Autodesk Fusion 360 part; units mm, degrees
sketch "Sketch1" plane through (0, 0, 0) normal (1, 0, 0) x (0, 1, 0) in component "latch_shuttle"
  arc A0 (-8.3077, 5.5575) -> (-1.6746, 2.5672) centre (9.4182, 36.0259) ccw
  arc A1 (-8.3077, 5.5575) -> (-9.6608, 5.2196) centre (-8.8106, 4.6931) ccw
  line L0 (-12.0836, 1.3076) -> (-9.6608, 5.2196)
  arc A2 (-12.0836, 1.3076) -> (-11.739, -0.0818) centre (-11.2334, 0.781) ccw
  arc A3 (-11.739, -0.0818) -> (-10.3245, -0.8742) centre (9.4182, 36.0259) ccw
  arc A4 (-10.3245, -0.8742) -> (-9.5002, -0.6041) centre (-10.0414, -0.3452) ccw
  line L1 (-9.5002, -0.6041) -> (-8.9235, 0.6015)
  arc A5 (-5.6086, 0.4414) -> (-8.9235, 0.6015) centre (-7.2997, -0.1753) ccw
  line L2 (-5.6086, 0.4414) -> (-4.4802, -2.6531)
  arc A6 (-4.4802, -2.6531) -> (-3.2044, -3.8747) centre (-2.6012, -1.9679) ccw
  arc A7 (-3.2044, -3.8747) -> (7.5742, -5.7831) centre (9.4182, 36.0259) ccw
  arc A8 (7.5742, -5.7831) -> (8.6182, -4.784) centre (7.6182, -4.784) ccw
  line L3 (8.6182, 3.9982) -> (8.6182, -4.784)
  arc A9 (8.6182, 3.9982) -> (7.6743, 4.9966) centre (7.6182, 3.9982) ccw
  arc A10 (5.7512, 5.1647) -> (7.6743, 4.9966) centre (9.4182, 36.0259) ccw
  arc A11 (5.7512, 5.1647) -> (4.8102, 4.7397) centre (5.6332, 4.1717) ccw
  arc A12 (-1.6746, 2.5672) -> (4.8102, 4.7397) centre (0.1191, 7.9776) ccw
extrude "Extrude1" add sketch "Sketch1" along normal mid plane 10.6 in component "latch_shuttle"
chamfer "Chamfer1" distance 0.4 angle 45 34 edges at (5.3, -5.0685, 3.8907) (5.3, -9.0529, 5.6633) (5.3, -10.8722, 3.2636) (5.3, -12.204, 0.5403) (5.3, -11.0356, -0.4848) (5.3, -9.8546, -0.9153) (5.3, -9.2118, -0.0013) (5.3, -7.2129, 1.6226) (5.3, -5.0444, -1.1058) (5.3, -3.9845, -3.4124) (5.3, 2.1222, -5.1828) (5.3, 8.3096, -5.5066) (5.3, 8.6182, -0.3929) (5.3, 8.3449, 4.6851) (5.3, 6.7115, 5.0657) (5.3, 5.2216, 5.0831) (5.3, 1.9298, 2.5728) (-5.3, 8.6182, -0.3929) (-5.3, 8.3096, -5.5066) (-5.3, 2.1222, -5.1828) (-5.3, -3.9845, -3.4124) (-5.3, -5.0444, -1.1058) (-5.3, -7.2129, 1.6226) (-5.3, -9.2118, -0.0013) (-5.3, -9.8546, -0.9153) (-5.3, -11.0356, -0.4848) (-5.3, -12.204, 0.5403) (-5.3, -10.8722, 3.2636) (-5.3, -9.0529, 5.6633) (-5.3, -5.0685, 3.8907) (-5.3, 1.9298, 2.5728) (-5.3, 5.2216, 5.0831) (-5.3, 6.7115, 5.0657) (-5.3, 8.3449, 4.6851) in component "latch_shuttle"
sketch "Sketch2" plane through (0, 8.6182, 0) normal (0, 1, 0) x (-1, 0, 0) in component "latch_shuttle"
  line L0 (4.9, -4.784) -> (4.9, 3.9982)
  line L1 (4.9, 3.9982) -> (-4.9, 3.9982)
  line L2 (-4.9, 3.9982) -> (-4.9, -4.784)
  line L3 (-4.9, -4.784) -> (4.9, -4.784)
  circle A0 centre (0, -0.4177) radius 1.6
  circle A1 centre (0, -0.4177) radius 2.35
extrude "Extrude2" cut sketch "Sketch2" against normal blind 4.2 contours A0 | A1 in component "latch_shuttle"
extrude "Extrude3" cut sketch "Sketch2" against normal blind 12 contours A0 in component "latch_shuttle"
component "latch_shuttle" placed x (1, 0, 0) y (0, 1, 0) z (0, 0, 1) at (0, 0, 0)
CAD build for the part. Positions are in the model's coordinates, mm. A direction names the side the tool comes from. Round coordinates to 2 decimals unless told otherwise and drop trailing zeros. Write each loop counter-clockwise with the first axis right and the second up, starting at its lowest first coordinate (ties: lowest second). Pieces come first, ordered by that corner, then holes.
Item 1: Tool access for faces 1 (the flat face through (5.1, -9.39, 0.09)), 2 (the cylindrical face through (-0.07, -5.02, 3.87)), 3 (the flat face through (-2, 4.418, -1)): list every direction of +Z, -Z, +X, -X, +Y, -Y with a clear straight run to the whole face (end or side of a thin tool).
Filled in:
face 1: -Z, +X
face 2: +Z, +X, -X
face 3: +Y
Item 2: Drop flat-ended pins along their axis: pin 1 Ø1.9 at (x, z) = (0, -0.42) entering from +Y; pin 2 Ø1.5 at (x, y) = (0, 1.5) entering from -Z; pin 3 Ø3 at (x, z) = (0, -0.42) entering from -Y; pin 4 Ø4 at (x, z) = (-4, -4) entering from -Y. Give the stop position or say it passes through.
Filled in:
pin 1: stops at y = -3.38
pin 2: stops at z = -5.21
pin 3: stops at y = -12.23
pin 4: stops at y = -4.72
Item 3: Band-saw the part on C-C on x = 0. Write the cut outline in (y, z), then the cut area to 3 significant figures.
Filled in:
outline: (-12.08, 1.31) arc R1 ccw to (-11.74, -0.08) arc R41.85 ccw to (-10.32, -0.87) arc R0.6 ccw to (-9.5, -0.6) - (-8.92, 0.6) arc R1.8 cw to (-5.61, 0.44) - (-4.48, -2.65) arc R2 ccw to (-3.2, -3.87) arc R41.85 ccw to (7.57, -5.78) arc R1 ccw to (8.62, -4.78) - (8.62, -2.77) - (4.42, -2.77) - (4.42, -2.02) - (-3.38, -2.02) - (-3.38, 1.18) - (4.42, 1.18) - (4.42, 1.93) - (8.62, 1.93) - (8.62, 4) arc R1 ccw to (7.67, 5) arc R31.08 cw to (5.75, 5.16) arc R1 ccw to (4.81, 4.74) arc R5.7 cw to (-1.67, 2.57) arc R35.25 cw to (-8.31, 5.56) arc R1 ccw to (-9.66, 5.22) - close
area: 97.5 mm2
Item 4: Band-saw the part on B-B on z = -1.75. Write the cut outline in (x, y).
Filled in:
outline: (-5.3, -4.38) - (-4.9, -4.81) - (4.9, -4.81) - (5.3, -4.38) - (5.3, 8.22) - (4.9, 8.62) - (1.94, 8.62) - (1.94, 4.42) - (0.89, 4.42) - (0.89, -3.38) - (-0.89, -3.38) - (-0.89, 4.42) - (-1.94, 4.42) - (-1.94, 8.62) - (-4.9, 8.62) - (-5.3, 8.22) - close
Item 5: Drill centre lines: L1, parallel to X at y = 3.25, z = -1.25; L2, parallel to Y at x = 4.5, z = 1; L3, parallel to Y at x = 1, z = 4.5. Where is each one in solid material? Low to high.
Filled in:
L1: x = -5.3 to -1.37, 1.37 to 5.3
L2: y = -12.21 to -8.66, -5.94 to 8.62
L3: y = -10.11 to -6.35, 4.64 to 8.48
Item 6: Band-saw the part on A-A on x = -4.5. Write the cut outline in (y, z), then the cut area to 3 significant figures.
Filled in:
outline: (-12.08, 1.31) arc R1 ccw to (-11.74, -0.08) arc R41.85 ccw to (-10.32, -0.87) arc R0.6 ccw to (-9.5, -0.6) - (-8.92, 0.6) arc R1.8 cw to (-5.61, 0.44) - (-4.48, -2.65) arc R2 ccw to (-3.2, -3.87) arc R41.85 ccw to (7.57, -5.78) arc R1 ccw to (8.62, -4.78) - (8.62, 4) arc R1 ccw to (7.67, 5) arc R31.08 cw to (5.75, 5.16) arc R1 ccw to (4.81, 4.74) arc R5.7 cw to (-1.67, 2.57) arc R35.25 cw to (-8.31, 5.56) arc R1 ccw to (-9.66, 5.22) - close
area: 142 mm2
Item 7: Mould opens along Y. For faces 4 (the cylindrical face through (0.21, 0.57, 1.17)), 5 (the flat face through (-2, 8.618, 2)), 6 (the flat face through (-0.069, -9.216, -0.01)) say: released by +Y, released by -Y, zero draft, split by the parting line, or undercut.
Filled in:
face 4: zero draft
face 5: released by +Y
face 6: undercut
